Check sheet for the modelled part. Datum: model origin and axes. Units: mm. A direction names the side the tool comes from. Give positions to 0.01 mm unless a question says otherwise; leave off trailing zeros. Order: outer loops, then holes, each group sorted by start corner. A loop starts at its lowest first (then second) coordinate and runs counter-clockwise, first axis right, second up. Notation, with made-up numbers: (27, -24.75) -> (50, -24.75) arc R15 cw to (50, -9.75) -> close; hole circle Ø3 at (43, -29). An arc over 180 degrees is marked (long way). One line per question, with ' | ' between items.
```python
from build123d import *

# Parameters (mm, degrees)
SALIENTE_EXTRUIR1_DEPTH = 10
CROQUIS1_3_W            = 698
CROQUIS1_3_H            = 90
SALIENTE_EXTRUIR2_DEPTH = 8
CROQUIS2_W              = 660
CROQUIS2_H              = 240
CORTAR_EXTRUIR1_DEPTH   = 10


with BuildPart() as part:
    # Croquis1 → Saliente-Extruir1 (new body)
    with BuildSketch(Plane(origin=(0, 0, 0), x_dir=(0, 0, -1), z_dir=(1, 0, 0))):
        Polygon((349, -45), (-349, -45), (-349.868447372, -45), (-349.868447372, -255), (350.131552628, -255), (350.131552628, -45), align=None)
    extrude(amount=SALIENTE_EXTRUIR1_DEPTH)

    # Croquis1<3> → Saliente-Extruir2 (add)
    with BuildSketch(Plane(origin=(0, 0, 0), x_dir=(0, 0, -1), z_dir=(1, 0, 0))):
        Rectangle(CROQUIS1_3_W, CROQUIS1_3_H)
    extrude(amount=SALIENTE_EXTRUIR2_DEPTH)

    # Croquis2 → Cortar-Extruir1 (cut)
    with BuildSketch(Plane.ZY):
        with Locations((-0.131552628, -105)):
            Rectangle(CROQUIS2_W, CROQUIS2_H)
    extrude(amount=-CORTAR_EXTRUIR1_DEPTH, mode=Mode.SUBTRACT)


solid = part.part
```
Q1. Thickness scan on line 1 (Y direction, x = 5, z = 217.5); line 2 (Z direction, x = 5, y = -54); line 3 (Z direction, x = 4.5, y = -44.5). Record the ranges inside material, lowest first.
Result sheet:
line 1: y = -255 to -225, 15 to 45 | line 2: z = -350.13 to -330.13, 329.87 to 349.87 | line 3: z = -349 to -330.13, 329.87 to 349
Q2. Section check A-A (y = -110). Enter the section's corners in (x, z), and give its area (3 significant figures).
Result sheet:
outline: (0, -350.13) -> (10, -350.13) -> (10, -330.13) -> (0, -330.13) -> close; (0, 329.87) -> (10, 329.87) -> (10, 349.87) -> (0, 349.87) -> close | area: 400 mm2
Q3. Depth check by flat-ended pin: pin 1 Ø2.5 at (x, y) = (5.5, -8.5) entering from +Z. Enter the tip coordinate at first touch or a pass-through.
Result sheet:
pin 1: stops at z = 349
Q4. Access from +Z, -Z, +X, -X, +Y, -Y to the whole of each face (thin tool, end or side, straight path). Record for faces 1 (the face through (8, 24, 2)), 2 (the face through (0, -227, 27)).
Result sheet:
face 1: +Z, -Z, +X, +Y | face 2: +Z, -Z, -X, +Y, -Y
Q5. Section check C-C (x = 5). Enter the section's corners in (y, z).
Result sheet:
outline: (-255, -350.13) -> (-45, -350.13) -> (-45, -349) -> (45, -349) -> (45, 349) -> (-45, 349) -> (-45, 349.87) -> (-255, 349.87) -> close; hole (-225, -330.13) -> (15, -330.13) -> (15, 329.87) -> (-225, 329.87) -> close
Q6. Section check B-B (z = 114). Enter the section's corners in (x, y), and give its area (3 significant figures).
Result sheet:
outline: (0, -255) -> (10, -255) -> (10, -225) -> (0, -225) -> close; (0, 15) -> (8, 15) -> (8, 45) -> (0, 45) -> close | area: 540 mm2
